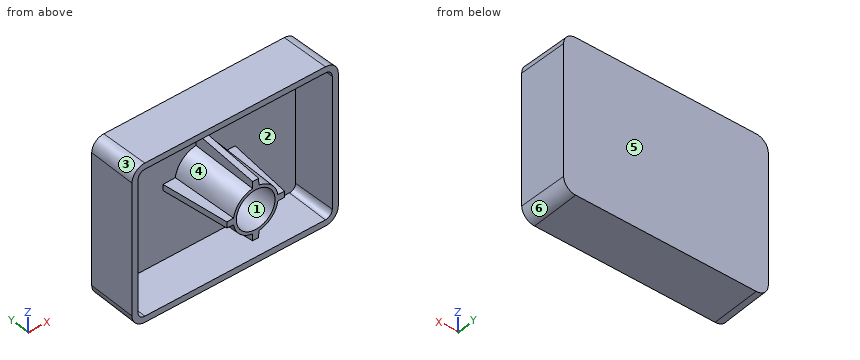
from build123d import *

# Parameters (mm, degrees)
BOSS_EXTRUDE1_DEPTH = 4
BOSS_EXTRUDE1_DRAFT = 1
SHELL1_T            = -0.5
SKETCH2_R           = 2
BOSS_EXTRUDE2_DEPTH = 5.5
BOSS_EXTRUDE2_TAPER = 1.5
CIRPATTERN1_COUNT   = 4
SKETCH4_R           = 1.605977431
CUT_EXTRUDE1_DEPTH  = 5.5
CUT_EXTRUDE1_DRAFT  = 1.5


with BuildPart() as part:
    # Sketch1 → Boss-Extrude1 (with draft: the straight prism first)
    with BuildSketch(Plane(origin=(0, 0, 0), x_dir=(1, 0, 0), z_dir=(0, 1, 0))):
        with BuildLine():
            Line((-7.5, -6.375), (7.5, -6.375))
            ThreePointArc((7.5, -6.375), (8.207106781, -6.082106781), (8.5, -5.375))
            Line((8.5, -5.375), (8.5, 5.375))
            ThreePointArc((8.5, 5.375), (8.207106781, 6.082106781), (7.5, 6.375))
            Line((7.5, 6.375), (-7.5, 6.375))
            ThreePointArc((-7.5, 6.375), (-8.207106781, 6.082106781), (-8.5, 5.375))
            Line((-8.5, 5.375), (-8.5, -5.375))
            ThreePointArc((-8.5, -5.375), (-8.207106781, -6.082106781), (-7.5, -6.375))
        make_face()
    extrude(amount=-BOSS_EXTRUDE1_DEPTH)
    # Boss-Extrude1: the draft: its side faces are tilted about the plane it starts from
    boss_extrude1_sides = [part.faces().sort_by_distance(p)[0] for p in [
        (0, -2, 6.375),
        (8.207106781, -2, 6.082106781),
        (8.5, -2, 0),
        (8.207106781, -2, -6.082106781),
        (0, -2, -6.375),
        (-8.207106781, -2, -6.082106781),
        (-8.5, -2, 0),
        (-8.207106781, -2, 6.082106781),
    ]]
    draft(boss_extrude1_sides, Plane(origin=(0, 0, 0), x_dir=(1, 0, 0), z_dir=(0, 1, 0)), BOSS_EXTRUDE1_DRAFT)

    # Shell1
    shell1_openings = [part.faces().sort_by_distance(p)[0] for p in [
        (0, -4, 0),
    ]]
    offset(amount=SHELL1_T, openings=shell1_openings, kind=Kind.INTERSECTION)

    # Sketch2 → Boss-Extrude2 (add)
    with BuildSketch(Plane.XZ.offset(0.5)):
        Circle(SKETCH2_R)
    extrude(amount=BOSS_EXTRUDE2_DEPTH, taper=BOSS_EXTRUDE2_TAPER)

    # Rib1: read off the stored shape, not the designer's step
    # Rib1: loft between two sections, ruled curve by curve
    rib1_from = [
        Edge.make_line((1.982008139, -0.5, 0.267663478), (3, -0.5, 0.25)),
        Edge.make_line((1.982008139, -0.5, -0.267663478), (3, -0.5, -0.25)),
        Edge.make_line((3, -0.5, -0.25), (3, -0.5, 0.25)),
        Edge.make_line((1.982008139, -0.5, -0.267663478), (1.982008139, -0.5, 0.267663478)),
    ]
    rib1_to = [
        Edge.make_line((1.837716138, -6, 0.259714502), (2.397587968, -6, 0.25)),
        Edge.make_line((1.837716138, -6, -0.259714502), (2.397587968, -6, -0.25)),
        Edge.make_line((2.397587968, -6, -0.25), (2.397587968, -6, 0.25)),
        Edge.make_line((1.837716138, -6, -0.259714502), (1.837716138, -6, 0.259714502)),
    ]
    rib1 = Solid(Shell([*[Face.make_surface_from_curves(rib1_from[k], rib1_to[k]) for k in range(4)], Face(Wire(rib1_from)), Face(Wire(rib1_to))]))
    add(rib1)

    # CirPattern1: Rib1 ×4 about axis
    cirpattern1_axis = Axis((0, 0, 0), (0, 1, 0))
    for i in range(1, CIRPATTERN1_COUNT):
        add(rib1.rotate(cirpattern1_axis, i * 360 / CIRPATTERN1_COUNT))


with BuildPart() as cut_extrude1_tool:
    # Sketch4 → Cut-Extrude1 (with draft: the straight prism first)
    with BuildSketch(Plane.XZ.offset(6)):
        Circle(SKETCH4_R)
    extrude(amount=-CUT_EXTRUDE1_DEPTH)
    # Cut-Extrude1: the draft: its side faces are tilted about the plane it starts from
    cut_extrude1_sides = [cut_extrude1_tool.faces().sort_by_distance(p)[0] for p in [
        (-1.605977431, -3.25, 0),
    ]]
    draft(cut_extrude1_sides, Plane.XZ.offset(6), CUT_EXTRUDE1_DRAFT)


with BuildPart() as part_1:
    add(part.part)

    # Cut-Extrude1: cut by cut_extrude1_tool
    add(cut_extrude1_tool.part, mode=Mode.SUBTRACT)


solid = part_1.part
Input: part model. Units: mm. Frame: model coordinates. Face numbers are marked on the shaded views. A direction names the side the tool comes from. Round coordinates to 2 decimals unless told otherwise and drop trailing zeros. Order: outer loops, then holes, each group sorted by start corner. A loop starts at its lowest first (then second) coordinate and runs counter-clockwise, first axis right, second up.
1. Set-up query: the marked faces 1, 2 and 3. Return all of +Z, -Z, +X, -X, +Y, -Y with unobstructed straight access to the full face (end or side cutting, diameter ignored); none if empty.
The answers:
face 1: none
face 2: -Y
face 3: +Z, -X, +Y
2. Cut plane C-C, the plane y = -3.75. State how many separate pieces and enclosed holes the cut face has, then the cut area to 3 significant figures.
The answers:
separate pieces: 2
enclosed holes: 2
area: 32.6 mm2
3. Pin query (flat end, axial travel): P1, Ø3, axis at x = 0.5, y = -2, coming from the +Z side; P2, Ø1.5, axis at x = -1.5, y = -1.5, coming from the -Z side. Return the tip coordinate at first contact, or that it passes through.
The answers:
P1: stops at z = 6.44
P2: stops at z = -6.41
4. Material intervals for line 1 (X direction, y = -3.75, z = 4.5); line 2 (X direction, y = -3.5, z = -1); line 3 (X direction, y = -2.5, z = -1), sorted ascending.
The answers:
line 1: x = -8.57 to -8.07, 8.07 to 8.57
line 2: x = -8.56 to -8.06, -1.64 to -1.34, 1.34 to 1.64, 8.06 to 8.56
line 3: x = -8.54 to -8.04, -1.67 to -1.37, 1.37 to 1.67, 8.04 to 8.54
5. Cut plane A-A, the plane z = -4.75. Output: boundary loops of the cut face in (x, y).
The answers:
outline: (-8.57, -4) - (-8.07, -4) - (-8.01, -0.5) - (8.01, -0.5) - (8.07, -4) - (8.57, -4) - (8.5, 0) - (-8.5, 0) - close
6. Cut plane B-B, the plane x = 5.25. Output: boundary loops of the cut face in (y, z) (3 decimals), then the cut area to 3 significant figures.
The answers:
outline: (-4, -6.445) - (0, -6.375) - (0, 6.375) - (-4, 6.445) - (-4, 5.945) - (-0.5, 5.884) - (-0.5, -5.884) - (-4, -5.945) - close
area: 9.88 mm2
7. Mould query, pull axis X, two halves, no side actions, for the marked faces 4, 5 and 6. Classes: released by +X, released by -X, zero draft, split by the parting line, or undercut.
The answers:
face 4: undercut
face 5: zero draft
face 6: released by +X
